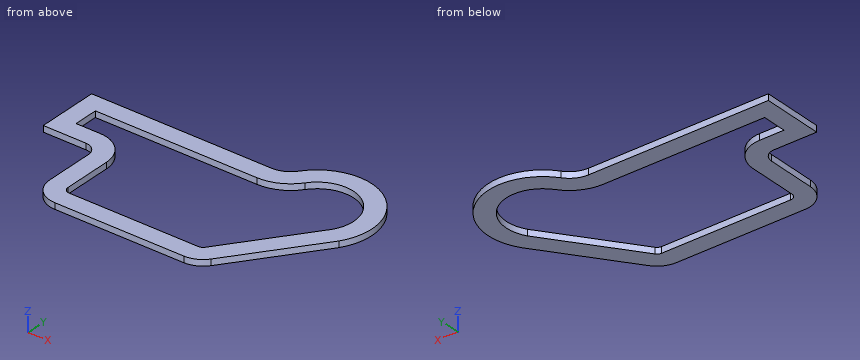
from build123d import *

# Parameters (mm, degrees)
BOSS_EXTRUDE1_DEPTH = 5


with BuildPart() as part:
    # Sketch2 → Boss-Extrude1 (new body)
    with BuildSketch(Plane.XY):
        with BuildLine():
            Line((0, 0), (0, 50))
            Line((0, 50), (147.694165659, 50))
            ThreePointArc((147.694165659, 50), (156.708879353, 52.146850782), (163.788268533, 58.126506299))
            ThreePointArc((163.788268533, 58.126506299), (225.679200393, 68.364882321), (237.666102591, 6.788702139))
            Line((237.666102591, 6.788702139), (187.081159294, -61.863810699))
            ThreePointArc((187.081159294, -61.863810699), (180, -67.850437165), (170.979917239, -70))
            Line((170.979917239, -70), (65, -70))
            ThreePointArc((65, -70), (50.857864376, -64.142135624), (45, -50))
            Line((45, -50), (45, -10))
            ThreePointArc((45, -10), (42.071067812, -2.928932188), (35, 0))
            Line((35, 0), (0, 0))
        make_face()
        with BuildLine():
            Line((15, 35), (147.694165659, 35))
            ThreePointArc((147.694165659, 35), (163.469914624, 38.756988868), (175.858845689, 49.221386023))
            ThreePointArc((175.858845689, 49.221386023), (216.96392633, 56.154330461), (225.315559898, 15.313865357))
            Line((225.315559898, 15.313865357), (175.005227753, -52.965952675))
            ThreePointArc((175.005227753, -52.965952675), (173.23493793, -54.462609291), (170.979917239, -55))
            Line((170.979917239, -55), (65, -55))
            ThreePointArc((65, -55), (61.464466094, -53.535533906), (60, -50))
            Line((60, -50), (60, -10))
            ThreePointArc((60, -10), (52.67766953, 7.67766953), (35, 15))
            Line((35, 15), (15, 15))
            Line((15, 15), (15, 35))
        make_face(mode=Mode.SUBTRACT)
    extrude(amount=BOSS_EXTRUDE1_DEPTH)


solid = part.part
The model under review builds one solid part; all positions refer to its coordinate system, in mm. Round coordinates to 2 decimals unless told otherwise and drop trailing zeros. Order: outer loops, then holes, each group sorted by start corner. A loop starts at its lowest first (then second) coordinate and runs counter-clockwise, first axis right, second up. Notation, with made-up numbers: (18.5, 82.25) -> (32.5, 82.25) arc R20 ccw to (32.5, 100.25) -> close; hole circle Ø11 at (69.25, 51.5). An arc over 180 degrees is marked (long way). Write item = value, one per line. Start each with the question number.
Item 1: Consider section A-A on z = 1.8. Write out the cut boundary in (x, y), plus the area to 3 significant figures.
Item 2: For line 1 along Y through (x, z) = (143, 0.25); line 2 along X through (y, z) = (31, 3.55); line 3 along Y through (x, z) = (50, 4.75), list the stretches that pass through material, from the lowest coordinate up.
Item 3: Consider section B-B on x = 200. Write out the cut boundary in (y, z).
Item 4: Consider section C-C on y = 39.5. Write out the cut boundary in (x, z), plus the area to 3 significant figures.
Item 5: Clearance check with flat-ended pins moving along their axes: pin 1 Ø1.5 at (y, z) = (22.5, 3.5) entering from +X; pin 2 Ø2.5 at (x, z) = (28.5, 2.5) entering from +Y; pin 3 Ø2.5 at (y, z) = (-23.5, 1.5) entering from +X. State where each tip first meets the part, or that it passes through.
Conclusion:
q1.outline = (0, 0) -> (35, 0) arc R10 cw to (45, -10) -> (45, -50) arc R20 ccw to (65, -70) -> (170.98, -70) arc R20 ccw to (187.08, -61.86) -> (237.67, 6.79) arc R45 ccw to (163.79, 58.13) arc R20 cw to (147.69, 50) -> (0, 50) -> close; hole (15, 15) -> (35, 15) arc R25 cw to (60, -10) -> (60, -50) arc R5 ccw to (65, -55) -> (170.98, -55) arc R5 ccw to (175.01, -52.97) -> (225.32, 15.31) arc R30 ccw to (175.86, 49.22) arc R35 cw to (147.69, 35) -> (15, 35) -> close
q1.area = 9,510 mm2
q2.line_1 = -70 to -55, 35 to 50
q2.line_2 = 0 to 15, 230 to 245
q2.line_3 = -63.23 to 10, 35 to 50
q3.outline = (-44.33, 0) -> (-19.04, 0) -> (-19.04, 5) -> (-44.33, 5) -> close; (61.41, 0) -> (76.41, 0) -> (76.41, 5) -> (61.41, 5) -> close
q4.outline = (0, 0) -> (164.86, 0) -> (164.86, 5) -> (0, 5) -> close; (228.89, 0) -> (244.27, 0) -> (244.27, 5) -> (228.89, 5) -> close
q4.area = 901 mm2
q5.pin_1 = 244.25
q5.pin_2 = 50
q5.pin_3 = 216.27
